from build123d import *

# Parameters (mm, degrees)
F0_R     = 1.85928
F1_DEPTH = 21.59
F2_R     = 1.07823
F3_DEPTH = 3.175
F4_W     = 20.6828571429
F4_H     = 24.13
F5_DEPTH = 12.7
F7_DEPTH = 4.445


# Not quite as in the source:
# - a feature names something its author has since deleted; it is built from what else it names


with BuildPart() as f1:
    # F0 (on Top) → F1 (new body)
    with BuildSketch(Plane.XY):
        Circle(F0_R)
    extrude(amount=-F1_DEPTH)

    # F2 (on Front) → F3 (cut, symmetric)
    with BuildSketch(Plane.XZ):
        with Locations((0, -2.7295311447)):
            Circle(F2_R)
    extrude(amount=F3_DEPTH, both=True, mode=Mode.SUBTRACT)

    # F4 (on Top) → F5 (join)
    with BuildSketch(Plane.XY):
        Rectangle(F4_W, F4_H)
    extrude(amount=F5_DEPTH)

    # F6 (on Front) → F7 (join, symmetric)
    with BuildSketch(Plane.XZ):
        Polygon((-9.8489131778, 4.8180790618), (-10.3458696976, 11.7754703388), (-23.9624772221, 10.8809489757), (-31.4168259501, 7.2034704499), (-36.187607795, 1.5381660778), (-38.076043129, -7.7052260749), (-34.7716075912, -8.3803259436), (-33.0594976471, 0), (-28.5344794393, 4.8180790618), (-21.7758696526, 4.8180790618), align=None)
    extrude(amount=F7_DEPTH, both=True)


solid = f1.part
Build history of the part. All positions in model axes, mm. A direction names the side the tool comes from. Coordinates: 2 decimals unless noted, no trailing zeros. Order: outer loops, then holes, each group sorted by start corner. A loop starts at its lowest first (then second) coordinate and runs counter-clockwise, first axis right, second up. Notation, with made-up numbers: (37, 77.5) - (92, 77.5) arc R15 ccw to (92, 86.5) - close; hole circle Ø4 at (-17, -5.75). An arc over 180 degrees is marked (long way). Put each result on its own line as item: value.
1. Saw through at B-B (y = 1). Write the cut outline in (x, z).
Answer sheet:
outline: (-38.08, -7.71) - (-34.77, -8.38) - (-33.06, 0) - (-28.53, 4.82) - (-10.34, 4.82) - (-10.34, 0) - (-1.57, 0) - (-1.57, -21.59) - (1.57, -21.59) - (1.57, 0) - (10.34, 0) - (10.34, 12.7) - (-10.34, 12.7) - (-10.34, 11.71) - (-10.35, 11.78) - (-23.96, 10.88) - (-31.42, 7.2) - (-36.19, 1.54) - close; hole circle Ø2.16 at (0, -2.73)
2. Saw through at C-C (z = 2.5). Write the cut outline in (x, y) (3 decimals), and give its area (3 significant figures).
Answer sheet:
outline: (-35.378, -4.445) - (-30.712, -4.445) - (-30.712, 4.445) - (-35.378, 4.445) - close; (-10.341, -12.065) - (10.341, -12.065) - (10.341, 12.065) - (-10.341, 12.065) - close
area: 541 mm^2
3. Saw through at A-A (x = 0). Write the cut outline in (y, z) (3 decimals), and give its area (3 significant figures).
Answer sheet:
outline: (-12.065, 0) - (-1.859, 0) - (-1.859, -1.651) - (1.859, -1.651) - (1.859, 0) - (12.065, 0) - (12.065, 12.7) - (-12.065, 12.7) - close; (-1.859, -21.59) - (1.859, -21.59) - (1.859, -3.808) - (-1.859, -3.808) - close
area: 379 mm^2
4. Drop flat-ended pins along their axis: P1, Ø5, axis at x = 2, z = -9, coming from the -Y side; P2, Ø12, axis at y = 4, z = 4, coming from the -X side; P3, Ø16, axis at x = -30, z = -1, coming from the +Y side (3 decimals). Give the stop position or say it passes through.
Answer sheet:
P1: stops at y = -1.86
P2: stops at x = -36.91
P3: stops at y = 4.445
5. Tool access for faces 1 (the face through (-24, -4.445, 5)), 2 (the face through (1.773, 0.558, -10.644)), 3 (the face through (-20, 0, 4.818)): list every direction of +Z, -Z, +X, -X, +Y, -Y with a clear straight run to the whole face (end or side of a thin tool).
Answer sheet:
face 1: +Z, -Z, -X, -Y
face 2: -Z
face 3: -Z, +Y, -Y
6. Saw through at D-D (z = -15). Write the cut outline in (x, y).
Answer sheet:
outline: circle Ø3.72 at (0, 0)
7. Probe line 1 along Z through (x, y) = (0, -1.05); line 2 along Y through (x, z) = (-12, 9) (3 decimals); line 3 along Z through (x, y) = (4, 10.25). List the from-to ranges inside material, lowest first. Write a range as [from, to].
Answer sheet:
line 1: z = [-21.59, -3.81], [-1.65, 12.7]
line 2: y = [-4.445, 4.445]
line 3: z = [0, 12.7]
8. Pull direction X, two halves, no side cores. Call faces 4 (the face through (0, 0, -21.59)), 5 (the face through (-10.341, 0, 3)), 6 (the face through (10.341, 0, 6)), 7 (the face through (-37.12, -0.06, -3.02)): pulls with the +X half, pulls with the -X half, needs draft (parallel to the pull), parting line crosses it, or undercut.
Answer sheet:
face 4: needs draft
face 5: undercut
face 6: pulls with the +X half
face 7: pulls with the -X half
